Input: part model. Units: mm. Frame: model coordinates. A direction names the side the tool comes from. Give positions to 0.01 mm unless a question says otherwise; leave off trailing zeros. Loops run counter-clockwise (first coordinate to the right, second up) from the corner with the lowest first, then second, coordinate; pieces in that order, holes last.
from build123d import *

# Parameters (mm, degrees)
SKETCH1_R               = 5
BOSS_EXTRUDE1_DEPTH     = 100
SKETCH2_R               = 11.5
BOSS_EXTRUDE2_DEPTH     = 5
SKETCH3_R               = 1.5
BOSS_EXTRUDE3_DEPTH     = 5
BOSS_EXTRUDE4_START     = 8
BOSS_EXTRUDE4_DEPTH     = 8
CUT_EXTRUDE2_DEPTH      = 8
CUT_EXTRUDE4_DEPTH      = 134.839635872
CUT_EXTRUDE4_DEPTH_BACK = 134.839635872
SKETCH7_W               = 13.423809299
SKETCH7_H               = 65.791523209
CUT_EXTRUDE5_DEPTH      = 48.105089111
CUT_EXTRUDE5_DEPTH_BACK = 48.105089111
SKETCH8_R               = 1.5
SKETCH9_R               = 5
SKETCH9_R_2             = 4.025
CUT_EXTRUDE6_DEPTH      = 25
FILLET1_R               = 10
BOSS_EXTRUDE5_START     = 25
SKETCH10_R              = 4.025
BOSS_EXTRUDE5_DEPTH     = 25
CUT_EXTRUDE7_DEPTH      = 10
SKETCH12_R              = 4.025
SKETCH12_R_2            = 4
CUT_EXTRUDE8_DEPTH      = 11
FILLET2_R               = 10
SKETCH13_R              = 4.105
SKETCH13_R_2            = 4.025
BOSS_EXTRUDE6_DEPTH     = 20
BOSS_EXTRUDE7_START     = 5
SKETCH14_R              = 4.105
BOSS_EXTRUDE7_DEPTH     = 5


with BuildPart() as part:
    # Sketch1 → Boss-Extrude1 (new body)
    with BuildSketch(Plane.XY):
        Circle(SKETCH1_R)
    extrude(amount=BOSS_EXTRUDE1_DEPTH)

    # Sketch2 → Boss-Extrude2 (add)
    with BuildSketch(Plane.XY.offset(100)):
        Circle(SKETCH2_R)
    extrude(amount=BOSS_EXTRUDE2_DEPTH)

    # Sketch3 → Boss-Extrude3 (add)
    with BuildSketch(Plane.XY.offset(105)):
        with Locations((8.302947015, 0)):
            Circle(SKETCH3_R)
    extrude(amount=BOSS_EXTRUDE3_DEPTH)

    # Sketch5 → Boss-Extrude4 (add)
    with BuildSketch(Plane(origin=(0, 0, 100), x_dir=(-1, 0, 0), z_dir=(0, 0, -1)).offset(BOSS_EXTRUDE4_START)):
        with BuildLine():
            Line((-10.45001903, 4.800739762), (0, 5))
            ThreePointArc((0, 5), (4.99977072, -0.04788268), (-0.095760969, -4.9990829))
            Line((-0.095760969, -4.9990829), (-10.45001903, -4.800739762))
            ThreePointArc((-10.45001903, -4.800739762), (-11.5, 0), (-10.45001903, 4.800739762))
        make_face()
    extrude(amount=-BOSS_EXTRUDE4_DEPTH)

    # Sketch6 → Cut-Extrude2 (cut)
    with BuildSketch(Plane(origin=(0, 0, 92), x_dir=(-1, 0, 0), z_dir=(0, 0, -1))):
        with BuildLine():
            ThreePointArc((-11.187749919, 2.661625773), (-11.326245042, 1.991525355), (-11.424640936, 1.314374177))
            ThreePointArc((-11.424640936, 1.314374177), (-10.141082355, 3.817380419), (-7.527110609, 4.856473577))
            Line((-7.527110609, 4.856473577), (-10.45001903, 4.800739762))
            ThreePointArc((-10.45001903, 4.800739762), (-10.871624232, 3.749371489), (-11.187749919, 2.661625773))
        make_face()
        with BuildLine():
            ThreePointArc((-11.424595573, -1.314768419), (-10.141131578, -3.817565911), (-7.527431975, -4.856723984))
            Line((-7.527431975, -4.856723984), (-10.45001903, -4.800739762))
            ThreePointArc((-10.45001903, -4.800739762), (-11.07531896, -3.09633815), (-11.424595573, -1.314768419))
        make_face()
    extrude(amount=-CUT_EXTRUDE2_DEPTH, mode=Mode.SUBTRACT)

    # Sketch7 → Cut-Extrude4 (cut, two sides: drawn at the far end of the back side and taken through both)
    with BuildSketch(Plane(origin=(-96.480203858, -4.620399557, 77.417416795), x_dir=(0.40721461787547164, -0.9133324996892062, 6.240488345448587e-15), z_dir=(0.9133324996892062, 0.40721461787547164, -3.9305527970726e-15)).offset(-CUT_EXTRUDE4_DEPTH_BACK)):
        with Locations((36.58009292, 44.521655191)):
            Rectangle(SKETCH7_W, SKETCH7_H)
    extrude(amount=CUT_EXTRUDE4_DEPTH + CUT_EXTRUDE4_DEPTH_BACK, mode=Mode.SUBTRACT)

    # Sketch8 → Cut-Extrude5 (cut, two sides: drawn at the far end of the back side and taken through both)
    with BuildSketch(Plane.XY.offset(110).offset(-CUT_EXTRUDE5_DEPTH_BACK)):
        with Locations((8.302947015, 0)):
            Circle(SKETCH8_R)
    extrude(amount=CUT_EXTRUDE5_DEPTH + CUT_EXTRUDE5_DEPTH_BACK, mode=Mode.SUBTRACT)

    # Sketch9 → Cut-Extrude6 (cut)
    with BuildSketch(Plane(origin=(0, 0, 65.791523209), x_dir=(-1, 0, 0), z_dir=(0, 0, -1))):
        with Locations(Location((0, 0, 0), (0, 0, 90))):
            Circle(SKETCH9_R)
        with Locations(Location((0, 0, 0), (0, 0, 90))):
            Circle(SKETCH9_R_2, mode=Mode.SUBTRACT)
    extrude(amount=-CUT_EXTRUDE6_DEPTH, mode=Mode.SUBTRACT)

    # Fillet1
    # the kernel refuses this fillet: 10 mm, written as the material it adds along each edge
    with BuildSketch(Plane(origin=(0, 0, 90.791523209), x_dir=(0, 1, 0), z_dir=(-1, 0, 0))) as fillet1_piece_1:
        with BuildLine():
            CenterArc((14.025, 4.306898536), FILLET1_R, 180, 25.511347951)
            Line((4.025, 4.306898536), (3.825, 4.306898536))
            Line((3.825, 4.306898536), (3.825, 0))
            Line((3.825, 0), (4.025, -0.2))
            ThreePointArc((4.025, -0.2), (4.5125, -0.2), (4.8195, -0.086137971))
            Line((4.8195, -0.086137971), (5, 0))
        make_face()
    revolve(axis=Axis((0, 0, 90.791523209), (0, 0, -1)))

    # Sketch10 → Boss-Extrude5 (add)
    with BuildSketch(Plane(origin=(0, 0, 65.791523209), x_dir=(-1, 0, 0), z_dir=(0, 0, -1)).offset(BOSS_EXTRUDE5_START)):
        with Locations(Location((0, 0, 0), (0, 0, 90))):
            Circle(SKETCH10_R)
    extrude(amount=-BOSS_EXTRUDE5_DEPTH)

    # Sketch11 → Cut-Extrude7 (cut)
    with BuildSketch(Plane(origin=(0, 0, 40.791523209), x_dir=(-1, 0, 0), z_dir=(0, 0, -1))):
        with BuildLine():
            Line((0, -4.025), (-3.918585251, 0.919409938))
            ThreePointArc((-3.918585251, 0.919409938), (-3.154461127, -2.5), (0, -4.025))
        make_face()
    extrude(amount=-CUT_EXTRUDE7_DEPTH, mode=Mode.SUBTRACT)

    # Sketch12 → Cut-Extrude8 (cut)
    with BuildSketch(Plane(origin=(0, 0, 40.791523209), x_dir=(-1, 0, 0), z_dir=(0, 0, -1))):
        with Locations(Location((0, 0, 0), (0, 0, 90))):
            Circle(SKETCH12_R)
        with Locations(Location((0, 0, 0), (0, 0, 90))):
            Circle(SKETCH12_R_2, mode=Mode.SUBTRACT)
    extrude(amount=-CUT_EXTRUDE8_DEPTH, mode=Mode.SUBTRACT)

    # Fillet2
    # the kernel refuses this fillet: 10 mm, written as the material it adds along each edge
    with BuildSketch(Plane(origin=(0, 0, 51.791523209), x_dir=(0, 1, 0), z_dir=(-1, 0, 0))) as fillet2_piece_1:
        with BuildLine():
            CenterArc((14, 0.706664701), FILLET2_R, 180, 4.052267945)
            Line((4, 0.706664701), (4, 0))
            Line((4, 0), (4.025, 0))
        make_face()
    revolve(axis=Axis((0, 0, 51.791523209), (0, 0, -1)))

    # Sketch13 → Boss-Extrude6 (add)
    with BuildSketch(Plane(origin=(0, 0, 72.432039474), x_dir=(-1, 0, 0), z_dir=(0, 0, -1))):
        with Locations(Location((0, 0, 0), (0, 0, 90))):
            Circle(SKETCH13_R)
        with Locations(Location((0, 0, 0), (0, 0, 90))):
            Circle(SKETCH13_R_2, mode=Mode.SUBTRACT)
    extrude(amount=-BOSS_EXTRUDE6_DEPTH)

    # Sketch14 → Boss-Extrude7 (add)
    with BuildSketch(Plane(origin=(0, 0, 72.432039474), x_dir=(-1, 0, 0), z_dir=(0, 0, -1)).offset(BOSS_EXTRUDE7_START)):
        with Locations(Location((0, 0, 0), (0, 0, 90))):
            Circle(SKETCH14_R)
    extrude(amount=-BOSS_EXTRUDE7_DEPTH)


solid = part.part
(1) Cut plane D-D (y = 6.5). Return the cut outline in (x, z).
Values follow:
outline: (-9.49, 100) - (9.49, 100) - (9.49, 105) - (-9.49, 105) - close
(2) Ray query, probe 1 along X at (y, z) = (0, 98.5); probe 2 along X at (y, z) = (0, 101); probe 3 along Y at (x, z) = (-0.25, 67). Return the intervals inside material, ascending.
Values follow:
probe 1: x = -5 to 6.8, 9.8 to 11.5
probe 2: x = -11.5 to 6.8, 9.8 to 11.5
probe 3: y = -4.02 to 4.02
(3) Mould query, pull axis Y, two halves, no side actions, for faces 1 (the cylindrical face through (-1.54, 3.72, 59.5)), 2 (the cylindrical face through (7.11, -0.91, 98.41)), 3 (the cylindrical face through (10.17, -3.79, 95.94)). Classes: +Y half, -Y half, draft (parallel to the pull), parting line (faces both ways), or undercut.
Values follow:
face 1: parting line
face 2: undercut
face 3: -Y half
(4) Reachability of faces 4 (the cylindrical face through (4.07, -0.53, 77.45)), 5 (the cylindrical face through (10.17, 3.79, 95.94)), 6 (the flat face through (2, -2, 50.792)), 7 (the flat face through (0, 0, 105)), 8 (the flat face through (0, 0, 40.792)) from +Z, -Z, +X, -X, +Y, -Y: full face, straight path, thin tool, end or side. Return the list, or none.
Values follow:
face 4: -Z
face 5: -Z, +X, +Y
face 6: -Z, +X, -Y
face 7: +Z, +X, -X, +Y, -Y
face 8: -Z, +X, -X, +Y, -Y
(5) Cut plane B-B (y = 0). Return the cut outline in (x, z) (3 decimals).
Values follow:
outline: (-11.5, 100) - (-5, 100) - (-5, 90.792) arc R10 cw to (-4.105, 87.747) - (-4.105, 67.432) - (-4.025, 67.432) - (-4.025, 51.792) arc R10 cw to (-4, 51.085) - (-4, 40.792) - (3.19, 40.792) - (3.19, 50.792) - (4, 50.792) - (4, 51.085) arc R10 cw to (4.025, 51.792) - (4.025, 67.432) - (4.105, 67.432) - (4.105, 87.747) arc R10 cw to (5, 90.792) - (5, 92) - (6.803, 92) - (6.803, 105) - (-11.5, 105) - close; (9.803, 92) - (11.5, 92) - (11.5, 105) - (9.803, 105) - close
(6) Pin query (flat end, axial travel): pin 1 Ø10 at (y, z) = (3, 74.5) entering from +X (3 decimals); pin 2 Ø12 at (y, z) = (9, 76) entering from -X; pin 3 Ø3 at (y, z) = (-4, 95) entering from -X. Return the tip coordinate at first contact, or that it passes through.
Values follow:
pin 1: stops at x = 4.105
pin 2: stops at x = -2.8
pin 3: stops at x = -4.33
(7) Cut plane A-A (x = 8.75). Return the cut outline in (y, z), and give its area (3 significant figures).
Values follow:
outline: (-7.46, 100) - (-4.64, 100) - (-4.64, 92) - (-1.43, 92) - (-1.43, 105) - (-7.46, 105) - close; (1.43, 92) - (4.64, 92) - (4.64, 100) - (7.46, 100) - (7.46, 105) - (1.43, 105) - close
area: 112 mm2
(8) Cut plane C-C (z = 59). Return the cut outline in (x, y) (3 decimals).
Values follow:
outline: circle Ø8.05 at (0, 0)
